```python
from build123d import *

# Parameters (mm, degrees)
F0_R     = 45
F0_W     = 5.2
F0_H     = 2.2
F1_DEPTH = 2
F2_R     = 1
F3_R     = 0.99999
F4_R     = 0.5


# Not quite as in the source:
# - a fillet or chamfer is up to 0.001 mm smaller than in the source, because OpenCascade refuses the exact size


with BuildPart() as f1:
    # F0 (on Top) → F1 (new body)
    with BuildSketch(Plane.XY):
        Circle(F0_R)
        Rectangle(F0_W, F0_H, mode=Mode.SUBTRACT)
    extrude(amount=F1_DEPTH)

    # F2
    f2_edges = [f1.edges().sort_by_distance(p)[0] for p in [
        (-45, 0, 2),
    ]]
    fillet(f2_edges, radius=F2_R)

    # F3 (radius 1 in the source; OpenCascade refuses exactly that, so slightly less here)
    f3_edges = [f1.edges().sort_by_distance(p)[0] for p in [
        (-45, 0, 0),
    ]]
    fillet(f3_edges, radius=F3_R)

    # F4
    f4_edges = [f1.edges().sort_by_distance(p)[0] for p in [
        (-2.6, 0, 0),
        (0, -1.1, 0),
        (2.6, 0, 0),
        (0, 1.1, 0),
    ]]
    fillet(f4_edges, radius=F4_R)


solid = f1.part
```
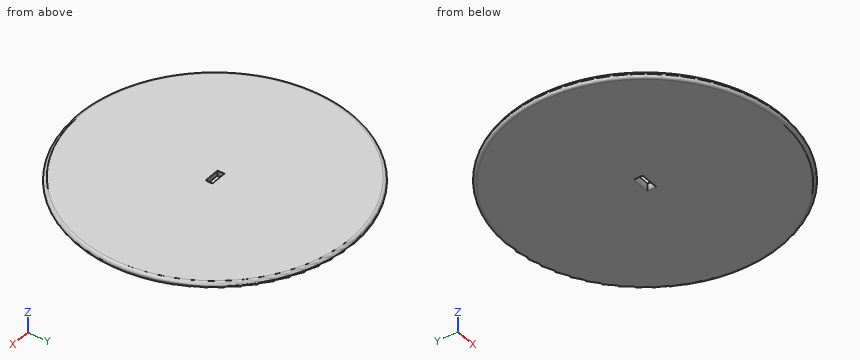
Could you check a few things on this model? Use its own coordinates, in mm. Round coordinates to 2 decimals unless told otherwise and drop trailing zeros. Loops run counter-clockwise (first coordinate to the right, second up) from the corner with the lowest first, then second, coordinate; pieces in that order, holes last. Notation, with made-up numbers: M 25,-10 L 47,-10 A14 ccw 47,13 Z; hole C 7.5,27.5 d1. An arc over 180 degrees is marked long. Answer as CSV lines item,"result".
1) Imagine slicing it at C-C on z = 1.45. List the corners of the cut face in (x, y) for me, and give its area (3 significant figures).
From the geometry:
outline,"C 0,0 d89.79; hole M -2.6,-1.1 L 2.6,-1.1 L 2.6,1.1 L -2.6,1.1 Z"
area,"6,320 mm^2"
2) For pin 1 Ø0.5 at (x, z) = (-1, 1.5) entering from +Y; pin 2 Ø0.5 at (x, z) = (0, 1) entering from -Y, each with a flat end and sliding along its axis, tell me the tip position at first contact or that it passes through.
From the geometry:
pin 1,"y = 44.96"
pin 2,"y = -45"
3) If I drill on probe 1 along X at (y, z) = (5.5, 1.6); probe 2 along Y at (x, z) = (3, 0.4); probe 3 along X at (y, z) = (-28.5, 1.2), over which ranges is the centre line in solid material (lowest first)?
From the geometry:
probe 1,"-44.46 to 44.46"
probe 2,"-44.7 to 44.7"
probe 3,"-34.8 to 34.8"
